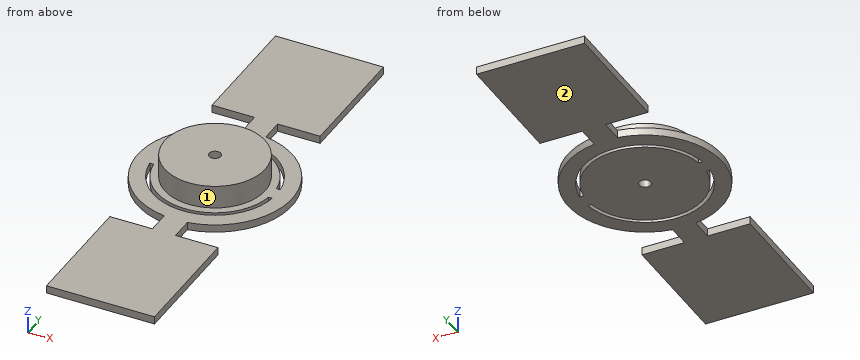
```python
from build123d import *

# Parameters (mm, degrees)
SKETCH043_R     = 6.5
PAD013_DEPTH    = 3
PAD014_DEPTH    = 1
SKETCH057_R     = 0.75
POCKET034_DEPTH = 5


with BuildPart() as part:
    # Sketch043 → Pad013 (new body)
    with BuildSketch(Plane.XY):
        Circle(SKETCH043_R)
    extrude(amount=PAD013_DEPTH)

    # Sketch044 (on Face2 of Pad013) → Pad014 (join)
    with BuildSketch(Plane(origin=(0, 0, 0), x_dir=(1, 0, 0), z_dir=(0, 0, -1))):
        with BuildLine():
            ThreePointArc((-1.5, 9.88686), (-10, 0), (-1.5, -9.88686))
            Line((-1.5, -9.88686), (-1.5, -12.88686))
            Line((-1.5, -12.88686), (-7, -12.88686))
            Line((-7, -12.88686), (-7, -28.88686))
            Line((-7, -28.88686), (7, -28.88686))
            Line((7, -28.88686), (7, -12.88686))
            Line((7, -12.88686), (1.5, -12.88686))
            Line((1.5, -9.88686), (1.5, -12.88686))
            ThreePointArc((1.5, -9.88686), (10, 0), (1.5, 9.88686))
            Line((1.5, 9.88686), (1.5, 12.88686))
            Line((7, 12.88686), (1.5, 12.88686))
            Line((7, 28.88686), (7, 12.88686))
            Line((-7, 28.88686), (7, 28.88686))
            Line((-7, 12.88686), (-7, 28.88686))
            Line((-1.5, 12.88686), (-7, 12.88686))
            Line((-1.5, 9.88686), (-1.5, 12.88686))
        make_face()
        with BuildLine():
            Line((-7.937254, -1), (-7.437254, -1))
            ThreePointArc((-7.437254, -1), (0, -7.504182), (7.437254, -1))
            Line((7.437254, -1), (7.937254, -1))
            ThreePointArc((-7.937254, -1), (0, -8), (7.937254, -1))
        make_face(mode=Mode.SUBTRACT)
        with BuildLine():
            Line((-7.437254, 1), (-7.937254, 1))
            ThreePointArc((7.937254, 1), (0, 8), (-7.937254, 1))
            Line((7.437254, 1), (7.937254, 1))
            ThreePointArc((7.437254, 1), (0, 7.504182), (-7.437254, 1))
        make_face(mode=Mode.SUBTRACT)
    extrude(amount=PAD014_DEPTH)

    # Sketch057 (on Face3 of Pad014) → Pocket034 (cut)
    with BuildSketch(Plane.XY.offset(3)):
        Circle(SKETCH057_R)
    extrude(amount=-POCKET034_DEPTH, mode=Mode.SUBTRACT)


with BuildPart() as part_1:
    # Body013 placement: moved
    add(part.part.moved(Location((198, 0, 0))))


solid = part_1.part
```
Work out the finished part from the listing and answer in its coordinate system (mm). Face numbers are marked on the shaded views. A direction names the side the tool comes from. Give positions to 0.01 mm unless a question says otherwise; leave off trailing zeros. Write each loop counter-clockwise with the first axis right and the second up, starting at its lowest first coordinate (ties: lowest second). Pieces come first, ordered by that corner, then holes. Notation, with made-up numbers: (73.5, 32.5) -> (118.5, 32.5) arc R15 ccw to (118.5, 47.5) -> close; hole circle Ø8 at (89.5, 0.25). An arc over 180 degrees is marked (long way). Write item = value, one per line.
Q1. Section B-B on y = 0 is taken. Determine the outline of the cut face in (x, z), and give its area (3 significant figures).
Computed values:
outline = (188, -1) -> (197.25, -1) -> (197.25, 3) -> (191.5, 3) -> (191.5, 0) -> (188, 0) -> close; (198.75, -1) -> (208, -1) -> (208, 0) -> (204.5, 0) -> (204.5, 3) -> (198.75, 3) -> close
area = 53.0 mm^2
Q2. Section D-D on y = 23.5 is taken. Determine the outline of the cut face in (x, z).
Computed values:
outline = (191, -1) -> (205, -1) -> (205, 0) -> (191, 0) -> close
Q3. Section A-A on x = 198 is taken. Determine the outline of the cut face in (y, z), and give its area (3 significant figures).
Computed values:
outline = (-28.89, -1) -> (-8, -1) -> (-8, 0) -> (-28.89, 0) -> close; (-7.5, -1) -> (-0.75, -1) -> (-0.75, 3) -> (-6.5, 3) -> (-6.5, 0) -> (-7.5, 0) -> close; (0.75, -1) -> (7.5, -1) -> (7.5, 0) -> (6.5, 0) -> (6.5, 3) -> (0.75, 3) -> close; (8, -1) -> (28.89, -1) -> (28.89, 0) -> (8, 0) -> close
area = 89.8 mm^2
Q4. A tool of negligible diameter and unlimited length cuts with its end or side. For the marked faces 1 and 2, from which of +Z, -Z, +X, -X, +Y, -Y can it reach the whole face along a straight path? Write none if from no direction.
Computed values:
face_1 = +Z
face_2 = -Z, +X, -X, +Y, -Y
Q5. Consider line 1 along Y through (x, z) = (198, 1.15); line 2 along Y through (x, z) = (200.25, -0.1); line 3 along Y through (x, z) = (191.25, -0.05). Determine where each line is inside the solid, lowest interval first.
Computed values:
line_1 = -6.5 to -0.75, 0.75 to 6.5
line_2 = -28.89 to -12.89, -9.74 to -7.68, -7.16 to 7.16, 7.68 to 9.74, 12.89 to 28.89
line_3 = -28.89 to -12.89, -7.38 to -4.29, -3.28 to 3.28, 4.29 to 7.38, 12.89 to 28.89
Q6. Flat-ended cylindrical pins translate along their axes: pin 1 Ø1.1 at (y, z) = (-19, -0.5) entering from -X; pin 2 Ø0.6 at (x, z) = (190.5, -0.5) entering from -Y; pin 3 Ø1.1 at (y, z) = (11.5, -0.5) entering from +X. Find the tip coordinate at first contact, or state that the pin passes through.
Computed values:
pin_1 = 191
pin_2 = -6.94
pin_3 = 199.5
Q7. Section C-C on x = 195.5 is taken. Determine the outline of the cut face in (y, z).
Computed values:
outline = (-28.89, -1) -> (-12.89, -1) -> (-12.89, 0) -> (-28.89, 0) -> close; (-9.68, -1) -> (-7.6, -1) -> (-7.6, 0) -> (-9.68, 0) -> close; (-7.08, -1) -> (7.08, -1) -> (7.08, 0) -> (6, 0) -> (6, 3) -> (-6, 3) -> (-6, 0) -> (-7.08, 0) -> close; (7.6, -1) -> (9.68, -1) -> (9.68, 0) -> (7.6, 0) -> close; (12.89, -1) -> (28.89, -1) -> (28.89, 0) -> (12.89, 0) -> close
